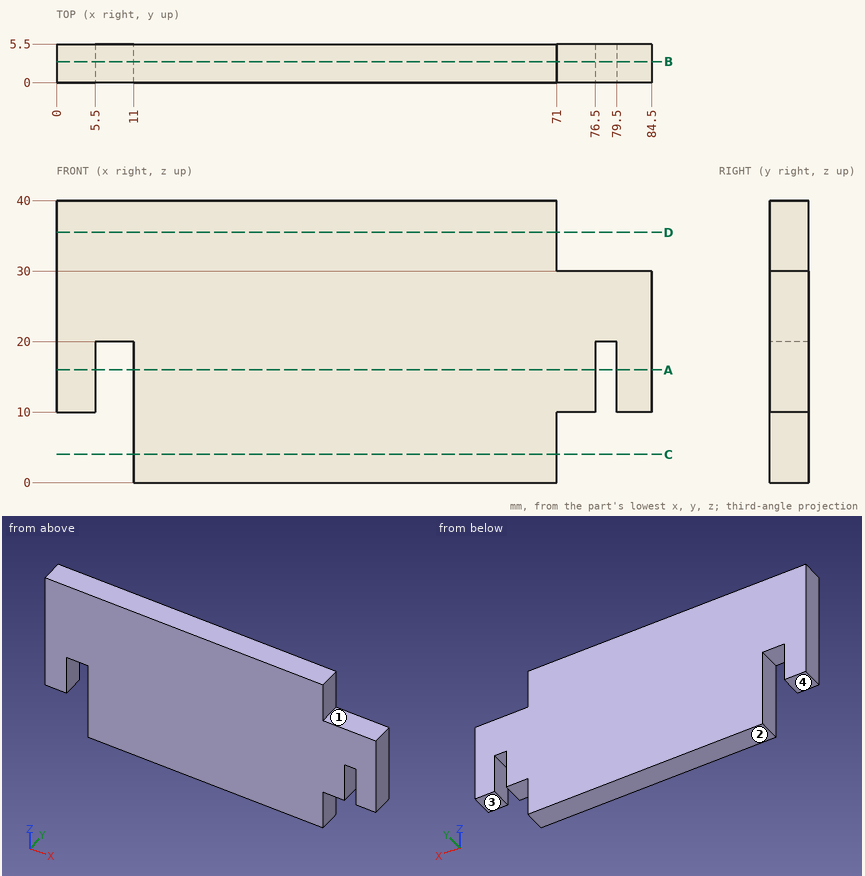
Part print with two shaded views. Sizes in mm from the minimum x, y, z corner. A direction names the side the tool comes from. Coordinates: 2 decimals unless noted, no trailing zeros. Write each loop counter-clockwise with the first axis right and the second up, starting at its lowest first coordinate (ties: lowest second). Pieces come first, ordered by that corner, then holes.
1. Drill centre lines: probe 1 along X at (y, z) = (4.75, 16); probe 2 along Z at (x, y) = (10.5, 1.3); probe 3 along X at (y, z) = (4.85, 8). Where is each one in solid material? Low to high.
Answer block:
probe 1: x = 0 to 5.5, 11 to 76.5, 79.5 to 84.5
probe 2: z = 20 to 40
probe 3: x = 11 to 71
2. Band-saw the part on B-B, the plane y = 3. Give the cut face in (x, z).
Answer block:
outline: (0, 10) - (5.5, 10) - (5.5, 20) - (11, 20) - (11, 0) - (71, 0) - (71, 10) - (76.5, 10) - (76.5, 20) - (79.5, 20) - (79.5, 10) - (84.5, 10) - (84.5, 30) - (71, 30) - (71, 40) - (0, 40) - close
3. Drop flat-ended pins along their axis: pin 1 (1.5 mm diameter, centred on x = 77.5, y = 2.5, fed in from -Z); pin 2 (4 mm diameter, centred on x = 46, z = 28, fed in from -Y); pin 3 (1.6 mm diameter, centred on x = 1.5, y = 4, fed in from -Z); pin 4 (1.6 mm diameter, centred on y = 1.5, z = 4, fed in from +X). Give the stop position or say it passes through.
Answer block:
pin 1: stops at z = 20
pin 2: stops at y = 0
pin 3: stops at z = 10
pin 4: stops at x = 71
4. Band-saw the part on D-D, the plane z = 35.5. Give the cut face in (x, y), and give its area (4 significant figures).
Answer block:
outline: (0, 0) - (71, 0) - (71, 5.5) - (0, 5.5) - close
area: 390.5 mm2
5. 3-axis set-ups, long thin cutter, end or side, ignore diameter. For the marked faces 1, 2, 3 and 4: which of +Z, -Z, +X, -X, +Y, -Y reach the whole face in a straight line?
Answer block:
face 1: +Z, +X, +Y, -Y
face 2: -Z, +X, -X, +Y, -Y
face 3: -Z, +X, +Y, -Y
face 4: -Z, -X, +Y, -Y
6. Band-saw the part on A-A, the plane z = 16. Give the cut face in (x, y), and give its area (3 significant figures).
Answer block:
outline: (0, 0) - (5.5, 0) - (5.5, 5.5) - (0, 5.5) - close; (11, 0) - (76.5, 0) - (76.5, 5.5) - (11, 5.5) - close; (79.5, 0) - (84.5, 0) - (84.5, 5.5) - (79.5, 5.5) - close
area: 418 mm2
7. Band-saw the part on C-C, the plane z = 4. Give the cut face in (x, y).
Answer block:
outline: (11, 0) - (71, 0) - (71, 5.5) - (11, 5.5) - close
